from build123d import *

# Parameters (mm, degrees)
BOSS_EXTRUDE1_DEPTH                                 = 10.1
SKETCH2_W                                           = 10.1
SKETCH2_H                                           = 2.668782353
BOSS_EXTRUDE2_DEPTH                                 = 11.626285019
BOSS_EXTRUDE3_DEPTH                                 = 4
SKETCH4_W                                           = 11.790327601
SKETCH4_H                                           = 5.654182735
BOSS_EXTRUDE4_DEPTH                                 = 10.1
CUT_EXTRUDE1_REACH                                  = 32.993
SKETCH6_W                                           = 5.300644637
SKETCH6_H                                           = 10.1
CBORE_FOR_4_BINDING_HEAD_MACHINE_SCREW1_D           = 3.4
CBORE_FOR_4_BINDING_HEAD_MACHINE_SCREW1_CBORE_D     = 6
CBORE_FOR_4_BINDING_HEAD_MACHINE_SCREW1_CBORE_DEPTH = 2.4
CBORE_FOR_4_BINDING_HEAD_MACHINE_SCREW2_D           = 3.4544
CBORE_FOR_4_BINDING_HEAD_MACHINE_SCREW2_CBORE_D     = 5.999999938
CBORE_FOR_4_BINDING_HEAD_MACHINE_SCREW2_CBORE_DEPTH = 2.400000026
FILLET1_R                                           = 2
FILLET2_R                                           = 3.2
FILLET3_R                                           = 5
CUT_EXTRUDE2_DEPTH                                  = 10.1


with BuildPart() as part:
    # Sketch1 → Boss-Extrude1 (new body)
    with BuildSketch(Plane.XY.offset(10.1)):
        with BuildLine():
            Line((8.423890913, 5.257630162), (8.423890913, -10.111152191))
            Line((8.423890913, -10.111152191), (10.022735266, -10.111152191))
            Line((10.022735266, -10.111152191), (21.064470639, 0.057225582))
            Line((21.064470639, 0.057225582), (21.064470639, 8.457630162))
            Line((21.064470639, 8.457630162), (5.223890913, 8.457630162))
            ThreePointArc((5.223890913, 8.457630162), (7.486632612, 7.520371862), (8.423890913, 5.257630162))
        make_face()
    extrude(amount=-BOSS_EXTRUDE1_DEPTH)

    # Sketch2 → Boss-Extrude2 (add)
    with BuildSketch(Plane.ZY.offset(-8.423890913)):
        with Locations((5.05, -8.776761014)):
            Rectangle(SKETCH2_W, SKETCH2_H)
    extrude(amount=BOSS_EXTRUDE2_DEPTH)

    # Sketch3 → Boss-Extrude3 (add)
    with BuildSketch(Plane(origin=(0, 0, 0), x_dir=(-1, 0, 0), z_dir=(0, 0, -1))):
        with BuildLine():
            Line((3.202394106, -10.111152191), (-10.022735266, -10.111152191))
            Line((-10.022735266, -10.111152191), (-21.064470639, 0.057225582))
            Line((-21.064470639, 0.057225582), (-21.064470639, 8.457630162))
            Line((-21.064470639, 8.457630162), (-5.223890913, 8.457630162))
            Line((-5.223890913, 8.457630162), (10.87546445, 10.911812897))
            Line((10.87546445, 10.911812897), (22.665792051, 10.911812897))
            Line((22.665792051, 10.911812897), (22.665792051, 5.257630162))
            ThreePointArc((22.665792051, 5.257630162), (15.602226067, -5.805749207), (3.202394106, -10.111152191))
        make_face()
    extrude(amount=BOSS_EXTRUDE3_DEPTH)

    # Sketch4 → Boss-Extrude4 (add)
    with BuildSketch(Plane.XY):
        with Locations((-16.77062825, 8.08472153)):
            Rectangle(SKETCH4_W, SKETCH4_H)
    extrude(amount=BOSS_EXTRUDE4_DEPTH)

    # Sketch6 → Cut-Extrude1 (cut, up to next)
    with BuildSketch(Plane(origin=(0, 8.457630162, 0), x_dir=(1, 0, 0), z_dir=(0, 1, 0)), mode=Mode.PRIVATE) as cut_extrude1_sk1:
        with Locations((-13.525786769, -5.05)):
            Rectangle(SKETCH6_W, SKETCH6_H)
    cut_extrude1_tool1 = extrude(cut_extrude1_sk1.sketch, amount=-CUT_EXTRUDE1_REACH, mode=Mode.PRIVATE) & part.part
    add(cut_extrude1_tool1.solids().sort_by_distance((-13.525787, 8.45763, 5.05))[0], mode=Mode.SUBTRACT)

    # CBORE for #4 Binding Head Machine Screw1 (through all)
    with Locations(Plane(origin=(0, 0, -4), x_dir=(-1, 0, 0), z_dir=(0, 0, -1))):
        with Locations((-5.423890913, -4.442369838)):
            CounterBoreHole(CBORE_FOR_4_BINDING_HEAD_MACHINE_SCREW1_D / 2, CBORE_FOR_4_BINDING_HEAD_MACHINE_SCREW1_CBORE_D / 2, CBORE_FOR_4_BINDING_HEAD_MACHINE_SCREW1_CBORE_DEPTH)

    # CBORE for #4 Binding Head Machine Screw2 (through all)
    with Locations(Plane(origin=(0, 0, -4), x_dir=(-1, 0, 0), z_dir=(0, 0, -1))):
        with Locations((17.076109087, 6.057630162)):
            CounterBoreHole(CBORE_FOR_4_BINDING_HEAD_MACHINE_SCREW2_D / 2, CBORE_FOR_4_BINDING_HEAD_MACHINE_SCREW2_CBORE_D / 2, CBORE_FOR_4_BINDING_HEAD_MACHINE_SCREW2_CBORE_DEPTH)

    # Fillet1
    fillet1_edges = [part.edges().sort_by_distance(p)[0] for p in [
        (-22.665792051, 10.911812897, 3.05),
    ]]
    fillet(fillet1_edges, radius=FILLET1_R)

    # Fillet2
    fillet2_edges = [part.edges().sort_by_distance(p)[0] for p in [
        (8.423890913, -7.442369838, 5.05),
    ]]
    fillet(fillet2_edges, radius=FILLET2_R)

    # Fillet3
    fillet3_edges = [part.edges().sort_by_distance(p)[0] for p in [
        (21.064470639, 0.057225582, 3.05),
        (10.022735266, -10.111152191, 3.05),
    ]]
    fillet(fillet3_edges, radius=FILLET3_R)

    # Sketch11 → Cut-Extrude2 (cut)
    with BuildSketch(Plane.XY.offset(10.1)):
        with BuildLine():
            Line((5.623890913, -7.442369838), (-20.076109087, -7.442369838))
            Line((-20.076109087, -7.442369838), (-20.076109087, 6.257630162))
            ThreePointArc((-20.076109087, 6.257630162), (-19.256008075, 8.23752915), (-17.276109087, 9.057630162))
            Line((-17.276109087, 9.057630162), (5.623890913, 9.057630162))
            ThreePointArc((5.623890913, 9.057630162), (7.6037899, 8.23752915), (8.423890913, 6.257630162))
            Line((8.423890913, 6.257630162), (8.423890913, -4.642369838))
            ThreePointArc((8.423890913, -4.642369838), (7.6037899, -6.622268825), (5.623890913, -7.442369838))
        make_face()
    extrude(amount=-CUT_EXTRUDE2_DEPTH, mode=Mode.SUBTRACT)


solid = part.part
Build history of the part. All positions in model axes, mm. A direction names the side the tool comes from. Coordinates: 2 decimals unless noted, no trailing zeros. Order: outer loops, then holes, each group sorted by start corner. A loop starts at its lowest first (then second) coordinate and runs counter-clockwise, first axis right, second up. Notation, with made-up numbers: (31, -9.5) - (68, -9.5) arc R19 ccw to (68, 3.5) - close; hole circle Ø9 at (4, -22.75). An arc over 180 degrees is marked (long way). Put each result on its own line as item: value.
1. Probe line 1 along X through (y, z) = (6, -0.5); line 2 along Z through (x, y) = (-15.5, 1.25); line 3 along Y through (x, z) = (-13, 6.75). List the from-to ranges inside material, lowest first. Write a range as [from, to].
Answer sheet:
line 1: x = [-22.67, -18.8], [-15.35, 21.06]
line 2: z = [-4, 0]
line 3: y = [9.06, 10.91]
2. Drop flat-ended pins along their axis: P1, Ø5, axis at y = -1, z = 3.5, coming from the -X side; P2, Ø4.5, axis at x = -17.08, y = 6.06, coming from the +Z side; P3, Ø3, axis at x = -13.5, z = 5, coming from the -Y side; P4, Ø1.8, axis at x = 5, y = -4, coming from the -Z side. Give the stop position or say it passes through.
Answer sheet:
P1: stops at x = 8.42
P2: stops at z = 0
P3: stops at y = 9.06
P4: passes through
3. Saw through at C-C (y = -0.25). Write the cut outline in (x, z).
Answer sheet:
outline: (-20.45, -4) - (20.39, -4) - (20.39, 10.1) - (8.42, 10.1) - (8.42, 0) - (-20.45, 0) - close
4. Saw through at A-A (z = 4.75). Write the cut outline in (x, y), and give its area (3 significant figures).
Answer sheet:
outline: (-22.67, 5.26) - (-20.08, 5.26) - (-20.08, 6.26) arc R2.8 cw to (-17.28, 9.06) - (-10.88, 9.06) - (-10.88, 10.91) - (-20.67, 10.91) arc R2 ccw to (-22.67, 8.91) - close; (-3.2, -10.11) - (8.07, -10.11) arc R5 ccw to (11.46, -8.79) - (19.45, -1.43) arc R5 ccw to (21.06, 2.25) - (21.06, 8.46) - (7.36, 8.46) arc R2.8 cw to (8.42, 6.26) - (8.42, -4.64) arc R2.8 cw to (5.62, -7.44) - (-3.2, -7.44) - close
area: 243 mm^2
5. Tool access for faces 1 (the face through (7.625, -6.6, 5.121)), 2 (the face through (-14, 9.058, 5)), 3 (the face through (-3.202, -9, 5)), 4 (the face through (-10.875, 10, 5)), 5 (the face through (-20.076, 6, 5)): list every direction of +Z, -Z, +X, -X, +Y, -Y with a clear straight run to the whole face (end or side of a thin tool).
Answer sheet:
face 1: +Z, -X
face 2: +Z, +X, -Y
face 3: +Z, -X, +Y, -Y
face 4: +Z, +X, +Y, -Y
face 5: +Z, -Y
6. Saw through at B-B (x = -16). Write the cut outline in (y, z), and give its area (3 significant figures).
Answer sheet:
outline: (-5.48, -4) - (3.26, -4) - (3.26, -1.6) - (4.71, -1.6) - (4.71, 0) - (-5.48, 0) - close; (7.41, -1.6) - (8.86, -1.6) - (8.86, -4) - (10.91, -4) - (10.91, 10.1) - (9.06, 10.1) - (9.06, 0) - (7.41, 0) - close
area: 66.5 mm^2
7. Pull direction Y, two halves, no side cores. Call faces 6 (the face through (15.4, -5.16, 3.15)), 7 (the face through (-19.938, 6.959, -2.817)), 8 (the face through (-18.45, 5.01, -0.79)), 9 (the face through (13, 8.458, 3)): pulls with the +Y half, pulls with the -Y half, needs draft (parallel to the pull), parting line crosses it, or undercut.
Answer sheet:
face 6: pulls with the -Y half
face 7: undercut
face 8: undercut
face 9: pulls with the +Y half
8. Saw through at D-D (x = 2). Write the cut outline in (y, z), and give its area (3 significant figures).
Answer sheet:
outline: (-10.11, -4) - (8.95, -4) - (8.95, 0) - (-7.44, 0) - (-7.44, 10.1) - (-10.11, 10.1) - close
area: 103 mm^2
